For this review, take the finished solid that the model builds, in its own axes (mm). Face numbers are marked on the shaded views. A direction names the side the tool comes from. Give positions to 0.01 mm unless a question says otherwise; leave off trailing zeros. Order: outer loops, then holes, each group sorted by start corner. A loop starts at its lowest first (then second) coordinate and runs counter-clockwise, first axis right, second up. Notation, with made-up numbers: (-7.5, -7) - (33.5, -7) arc R14 ccw to (33.5, 1) - close; hole circle Ø5 at (-0.5, 86.25). An arc over 180 degrees is marked (long way). Put each result on its own line as item: value. Start each with the question number.
Autodesk Inventor part; units mm, degrees
ref_plane "YZ Plane" through (0, 0, 0) normal (1, 0, 0) x (0, 1, 0)
ref_plane "XZ Plane" through (0, 0, 0) normal (0, 1, 0) x (-1, 0, 0)
ref_plane "XY Plane" through (0, 0, 0) normal (0, 0, 1) x (1, 0, 0)
sketch "Sketch1" plane through (0, 0, 0) normal (0, 0, 1) x (1, 0, 0)
  line L0 (0, 0) -> (-25.5293, 0)
  line L1 (-25.5293, 0) -> (-25.5293, 7.9022)
  line L2 (-25.5293, 7.9022) -> (-10.9446, 7.9022)
  line L3 (-10.9446, 7.9022) -> (-10.9446, 28.9877)
  line L4 (0, -5.7975) -> (0, 34.7852)
  line L5 (0, 0) -> (25.5293, 0)
  line L6 (25.5293, 0) -> (25.5293, 7.9022)
  line L7 (25.5293, 7.9022) -> (10.9446, 7.9022)
  line L8 (10.9446, 7.9022) -> (10.9446, 28.9877)
  line L9 (10.9446, 28.9877) -> (-10.9446, 28.9877)
extrude "Extrusion1" add sketch "Sketch1" along normal mid plane 20.32
sketch "Sketch2" plane through (0, 0, 10.16) normal (0, 0, 1) x (1, 0, 0)
  line L0 (-10.9446, 7.9022) -> (-25.5293, 7.9022)
  line L1 (-25.5293, 7.9022) -> (-25.5293, 0)
  line L2 (-25.5293, 0) -> (25.5293, 0)
  line L3 (25.5293, 0) -> (25.5293, 7.9022)
  line L4 (25.5293, 7.9022) -> (10.9446, 7.9022)
  line L5 (10.9446, 7.9022) -> (10.9446, 28.9877)
  line L6 (10.9446, 28.9877) -> (-10.9446, 28.9877)
  line L7 (-10.9446, 28.9877) -> (-10.9446, 7.9022)
  line L8 (0, -6.2231) -> (0, 37.3386)
  line L9 (0, 25.2482) -> (7.2771, 21.0468)
  line L10 (7.2771, 21.0468) -> (7.2771, 12.6439)
  line L11 (7.2771, 12.6439) -> (0, 8.4425)
  line L12 (0, 8.4425) -> (-7.2771, 12.6439)
  line L13 (-7.2771, 12.6439) -> (-7.2771, 21.0468)
  line L14 (-7.2771, 21.0468) -> (0, 25.2482)
  circle A0 centre (0, 16.8453) radius 4.8006
  point P0 (0, 0)
  dimension "d5" = 14.5542
  dimension "d6" = 9.6012
extrude "Extrusion2" cut sketch "Sketch2" against normal through all contours A0 L8 | L8 A0
extrude "Extrusion3" cut sketch "Sketch2" against normal blind 10.16 contours L9 L10 L11 L8 A0 | L8 A0 L12 L13 L14
sketch "Sketch3" plane through (-25.5293, 7.9022, 10.16) normal (0, 1, 0) x (1, 0, 0)
  line L0 (0, 20.32) -> (0, 0)
  line L1 (14.5848, 0) -> (0, 0)
  line L2 (14.5848, 20.32) -> (14.5848, 0)
  line L3 (0, 20.32) -> (14.5848, 20.32)
  line L4 (36.4739, 20.32) -> (36.4739, 0)
  line L5 (51.0586, 0) -> (36.4739, 0)
  line L6 (51.0586, 20.32) -> (51.0586, 0)
  line L7 (36.4739, 20.32) -> (51.0586, 20.32)
  circle A0 centre (9.0193, 10.16) radius 4.0005
  line L8 (14.5848, 20.32) -> (14.5848, 0)
  line L9 (36.4739, 0) -> (14.5848, 0)
  line L10 (36.4739, 20.32) -> (36.4739, 0)
  line L11 (14.5848, 20.32) -> (36.4739, 20.32)
  line L12 (25.5293, 24.384) -> (25.5293, -4.064)
  circle A1 centre (42.0393, 10.16) radius 4.0005
  point P0 (25.5293, 10.16)
  point P1 (0, 10.16)
  dimension "d11" = 8.001
  dimension "d15" = 33.02
extrude "Extrusion4" cut sketch "Sketch3" against normal through all contours A0 | A1
properties part number "y_axis_lead_screw_insert"
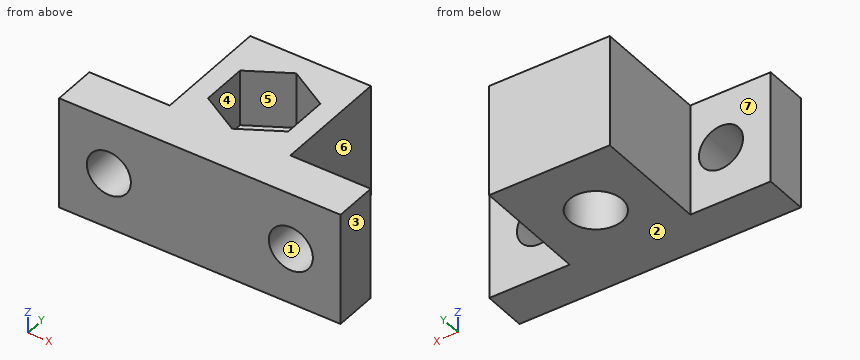
1. Add section A-A, the plane x = -16.51. Give the boundary of the cut face in (y, z).
2. Clearance check with flat-ended pins moving along their axes: pin 1 (4 mm diameter, centred on y = 16.5, z = 5.5, fed in from +X); pin 2 (10 mm diameter, centred on x = 17, z = 4, fed in from +Y); pin 3 (10 mm diameter, centred on y = 13.5, z = -0.5, fed in from -X). State where each tip first meets the part, or that it passes through.
3. Add section D-D, the plane y = 19.5. Give the boundary of the cut face in (x, z).
4. Tool access review of the marked faces 5, 6 and 7: name each direction out of +Z, -Z, +X, -X, +Y, -Y from which nothing blocks a thin tool from reaching the whole face with its end or side.
5. The part is to be moulded in two halves that separate along X. For the marked faces 1, 2, 3 and 4, say which applies: released by +X, released by -X, zero draft, split by the parting line, or undercut.
6. Wall thickness on line 1 (X direction, y = 4.25, z = 0); line 2 (Z direction, x = -16.51, y = 2); line 3 (Y direction, x = 0, z = -4.75): over which ranges is each line inside the solid? List them lowest first. Write a range as from..to.
7. Add section B-B, the plane z = 5. Give the boundary of the cut face in (x, y), then the cut area to 3 significant figures.
8. Add section C-C, the plane y = 6. Give the boundary of the cut face in (x, z), then the cut area to 3 significant figures.
Found:
1. outline: (0, -10.16) - (7.9, -10.16) - (7.9, -4) - (0, -4) - close; (0, 4) - (7.9, 4) - (7.9, 10.16) - (0, 10.16) - close
2. pin 1: stops at x = 10.94
2. pin 2: stops at y = 7.9
2. pin 3: stops at x = -10.94
3. outline: (-10.94, -10.16) - (-4, -10.16) - (-4, 0) - (-7.28, 0) - (-7.28, 10.16) - (-10.94, 10.16) - close; (4, -10.16) - (10.94, -10.16) - (10.94, 10.16) - (7.28, 10.16) - (7.28, 0) - (4, 0) - close
4. face 5: +Z
4. face 6: +Z, -Z, +X, +Y
4. face 7: +Z, -Z, -X, +Y
5. face 1: undercut
5. face 2: zero draft
5. face 3: released by +X
5. face 4: undercut
6. line 1: x = -25.53..-20.51, -12.51..12.51, 20.51..25.53
6. line 2: z = -10.16..-4, 4..10.16
6. line 3: y = 0..12.04, 21.65..28.99
7. outline: (-25.53, 0) - (25.53, 0) - (25.53, 7.9) - (10.94, 7.9) - (10.94, 28.99) - (-10.94, 28.99) - (-10.94, 7.9) - (-25.53, 7.9) - close; hole (-7.28, 12.64) - (0, 8.44) - (7.28, 12.64) - (7.28, 21.05) - (0, 25.25) - (-7.28, 21.05) - close
7. area: 682 mm^2
8. outline: (-25.53, -10.16) - (25.53, -10.16) - (25.53, 10.16) - (-25.53, 10.16) - close; hole circle Ø8 at (-16.51, 0); hole circle Ø8 at (16.51, 0)
8. area: 937 mm^2
